```python
from build123d import *

# Parameters (mm, degrees)
BOSS_EXTRUDE1_DEPTH = 7.5
SKETCH2_R           = 2
CUT_EXTRUDE1_DEPTH  = 58.68
CUT_EXTRUDE2_REACH  = 77.574
SKETCH3_R           = 1.05
FILLET1_R           = 2


with BuildPart() as part:
    # Sketch1 → Boss-Extrude1 (new, symmetric)
    with BuildSketch(Plane(origin=(0, 0, 0), x_dir=(0, 0, -1), z_dir=(1, 0, 0))):
        Polygon((0, 0), (0, 8), (25, 8), (40, -10), (40, -55.68), (20, -55.68), (20, 0), align=None)
    extrude(amount=BOSS_EXTRUDE1_DEPTH, both=True)

    # Sketch2 → Cut-Extrude1 (cut)
    with BuildSketch(Plane(origin=(0, 8, 0), x_dir=(1, 0, 0), z_dir=(0, 1, 0))):
        with Locations(Location((-4, 31, 0), (0, 0, 270))):
            Circle(SKETCH2_R)
        with Locations(Location((4, 31, 0), (0, 0, 270))):
            Circle(SKETCH2_R)
    extrude(amount=-CUT_EXTRUDE1_DEPTH, mode=Mode.SUBTRACT)

    # Sketch3 → Cut-Extrude2 (cut, up to next)
    with BuildSketch(Plane(origin=(0, 8, 0), x_dir=(1, 0, 0), z_dir=(0, 1, 0)), mode=Mode.PRIVATE) as cut_extrude2_sk1:
        with Locations(Location((-4, 31, 0), (0, 0, 270))):
            Circle(SKETCH3_R)
    cut_extrude2_tool1 = extrude(cut_extrude2_sk1.sketch, amount=-CUT_EXTRUDE2_REACH, mode=Mode.PRIVATE) & part.part
    # Sketch3 → Cut-Extrude2 (cut, up to next)
    with BuildSketch(Plane(origin=(0, 8, 0), x_dir=(1, 0, 0), z_dir=(0, 1, 0)), mode=Mode.PRIVATE) as cut_extrude2_sk2:
        with Locations(Location((4, 31, 0), (0, 0, 270))):
            Circle(SKETCH3_R)
    cut_extrude2_tool2 = extrude(cut_extrude2_sk2.sketch, amount=-CUT_EXTRUDE2_REACH, mode=Mode.PRIVATE) & part.part
    add(cut_extrude2_tool1.solids().sort_by_distance((-4, 8, -31))[0], mode=Mode.SUBTRACT)
    add(cut_extrude2_tool2.solids().sort_by_distance((4, 8, -31))[0], mode=Mode.SUBTRACT)

    # Fillet1
    fillet1_edges = [part.edges().sort_by_distance(p)[0] for p in [
        (0, 0, 0),
        (0, 8, 0),
        (0, 8, -25),
        (0, -10, -40),
        (0, 0, -20),
    ]]
    fillet(fillet1_edges, radius=FILLET1_R)


solid = part.part
```
CAD build for the part. Positions are in the model's coordinates, mm. A direction names the side the tool comes from. Round coordinates to 2 decimals unless told otherwise and drop trailing zeros. Write each loop counter-clockwise with the first axis right and the second up, starting at its lowest first coordinate (ties: lowest second). Pieces come first, ordered by that corner, then holes. Notation, with made-up numbers: (38, 4) -> (54, 4) arc R30 cw to (54, 43) -> close; hole circle Ø3 at (-31, 81.5). An arc over 180 degrees is marked (long way). Answer in a Markdown table with one row per item. Add a question column.
Item 1: Mould opens along X. For faces 4 (the face through (3, -50.68, -30)), 5 (the face through (0, -33, -40)), 6 (the face through (7.5, -23, -25)) say: pulls with the +X half, pulls with the -X half, needs draft (parallel to the pull), parting line crosses it, or undercut.
Item 2: Drill centre lines: line 1 (X direction, y = -16, z = -31); line 2 (Z direction, x = -4.25, y = -17.5); line 3 (Z direction, x = -5.5, y = -50). Where is each one in solid material? Low to high. Write a range as from..to.
Item 3: Which spindle directions (+Z, -Z, +X, -X, +Y, -Y) get a long thin tool onto all of the face, cutting with end or side? Do faces 1 (the face through (0, 0, -10)), 2 (the face through (-3.399, -23.363, -29.092)), 3 (the face through (-3.11, -53.14, -30.44)). Say none if no direction does.
Item 4: Saw through at C-C, the plane y = -41. Write the cut outline in (x, z).
Item 5: Saw through at D-D, the plane x = -0.5. Write the cut outline in (y, z).
Item 6: Saw through at B-B, the plane z = -31. Write the cut outline in (x, y), then the cut area to 3 significant figures.
Item 7: Saw through at A-A, the plane x = -4. Write the cut outline in (y, z), then the cut area to 3 significant figures.
Item 8: Drop flat-ended pins along their axis: pin 1 Ø5 at (x, y) = (-2.5, -29) entering from +Z; pin 2 Ø4.5 at (x, z) = (5, -30.5) entering from +Y; pin 3 Ø6.5 at (x, z) = (-4, -31) entering from +Y. Give the stop position or say it passes through.
Findings below:
| question | item | result |
|---|---|---|
| 1 | face 4 | undercut |
| 1 | face 5 | needs draft |
| 1 | face 6 | pulls with the +X half |
| 2 | line 1 | x = -7.5..-6, -2..2, 6..7.5 |
| 2 | line 2 | z = -40..-32.98, -29.02..-20 |
| 2 | line 3 | z = -40..-32.32, -29.68..-20 |
| 3 | face 1 | +Z, +X, -X, -Y |
| 3 | face 2 | +Y |
| 3 | face 3 | +Y, -Y |
| 4 | outline | (-7.5, -40) -> (7.5, -40) -> (7.5, -20) -> (-7.5, -20) -> close; hole circle Ø4 at (-4, -31); hole circle Ø4 at (4, -31) |
| 5 | outline | (-55.68, -40) -> (-10.72, -40) arc R2 ccw to (-9.44, -39.54) -> (7.28, -25.6) arc R2 ccw to (8, -24.06) -> (8, -2) arc R2 ccw to (6, 0) -> (2, 0) arc R2 ccw to (0, -2) -> (0, -18) arc R2 cw to (-2, -20) -> (-55.68, -20) -> close |
| 6 | outline | (-7.5, -55.68) -> (-5.05, -55.68) -> (-5.05, -50.68) -> (-6, -50.68) -> (-6, 0.8) -> (-7.5, 0.8) -> close; (-2.95, -55.68) -> (2.95, -55.68) -> (2.95, -50.68) -> (2, -50.68) -> (2, 0.8) -> (-2, 0.8) -> (-2, -50.68) -> (-2.95, -50.68) -> close; (5.05, -55.68) -> (7.5, -55.68) -> (7.5, 0.8) -> (6, 0.8) -> (6, -50.68) -> (5.05, -50.68) -> close |
| 6 | area | 414 mm^2 |
| 7 | outline | (-55.68, -40) -> (-10.72, -40) arc R2 ccw to (-9.44, -39.54) -> (-1.6, -33) -> (-50.68, -33) -> (-50.68, -32.05) -> (-55.68, -32.05) -> close; (-55.68, -29.95) -> (-50.68, -29.95) -> (-50.68, -29) -> (3.2, -29) -> (7.28, -25.6) arc R2 ccw to (8, -24.06) -> (8, -2) arc R2 ccw to (6, 0) -> (2, 0) arc R2 ccw to (0, -2) -> (0, -18) arc R2 cw to (-2, -20) -> (-55.68, -20) -> close |
| 7 | area | 1,080 mm^2 |
| 8 | pin 1 | stops at z = -20 |
| 8 | pin 2 | stops at y = 4.1 |
| 8 | pin 3 | stops at y = 4.7 |
